from build123d import *

# Parameters (mm, degrees)
SKETCH_1_W      = 16.3
SKETCH_1_H      = 18
EXTRUDE_1_DEPTH = 10
SKETCH_3_R      = 4
EXTRUDE_2_DEPTH = 12


with BuildPart() as part:
    # Эскиз1 → Бобышка-Вытянуть1 (new body)
    with BuildSketch(Plane(origin=(0, 0, 0), x_dir=(1, 0, 0), z_dir=(0, 1, 0))):
        with Locations((8.15, 9)):
            Rectangle(SKETCH_1_W, SKETCH_1_H)
    extrude(amount=EXTRUDE_1_DEPTH)

    # Эскиз3 → Бобышка-Вытянуть2 (add)
    with BuildSketch(Plane.XZ):
        with Locations(Location((8.15, -6, 0), (0, 0, 270))):
            Circle(SKETCH_3_R)
    extrude(amount=EXTRUDE_2_DEPTH)


solid = part.part
Verification items for the finished model (mm, model axes). A direction names the side the tool comes from. Coordinates: 2 decimals unless noted, no trailing zeros. Order: outer loops, then holes, each group sorted by start corner. A loop starts at its lowest first (then second) coordinate and runs counter-clockwise, first axis right, second up. Notation, with made-up numbers: (46, 25.25) -> (104, 25.25) arc R20 ccw to (104, 56.25) -> close; hole circle Ø2 at (-5.75, 67). An arc over 180 degrees is marked (long way). Put each result on its own line as item: value. Start each with the question number.
1. Cross-section at A-A, the plane x = 8.15. Record the boundary of the cut face in (y, z).
2. Cross-section at D-D, the plane x = 2.5. Record the boundary of the cut face in (y, z), then the cut area to 3 significant figures.
3. Access from +Z, -Z, +X, -X, +Y, -Y to the whole of each face (thin tool, end or side, straight path). Record for faces 1 (the flat face through (8, -12, -6)), 2 (the cylindrical face through (12.116, -5.916, -5.479)).
4. Cross-section at C-C, the plane y = -6.5. Record the boundary of the cut face in (x, z), then the cut area to 3 significant figures.
5. Material ranges on L1, parallel to Y at x = 11.5, z = -13.25; L2, parallel to Z at x = 10, y = -6.75; L3, parallel to Z at x = 11.25, y = -5.75, recorded low to high. Write a range as [from, to].
6. Cross-section at B-B, the plane z = -6. Record the boundary of the cut face in (x, y), then the cut area to 3 significant figures.
7. Go/stop test with a flat-tipped pin: pin 1 Ø3 at (y, z) = (-7, -7.5) entering from +X. Record where the tip stops, or that it passes through.
Computed:
1. outline: (-12, -10) -> (0, -10) -> (0, -18) -> (10, -18) -> (10, 0) -> (0, 0) -> (0, -2) -> (-12, -2) -> close
2. outline: (0, -18) -> (10, -18) -> (10, 0) -> (0, 0) -> close
2. area: 180 mm2
3. face 1: +Z, -Z, +X, -X, -Y
3. face 2: -Y
4. outline: circle Ø8 at (8.15, -6)
4. area: 50.3 mm2
5. L1: [0, 10]
5. L2: [-9.55, -2.45]
5. L3: [-8.53, -3.47]
6. outline: (0, 0) -> (4.15, 0) -> (4.15, -12) -> (12.15, -12) -> (12.15, 0) -> (16.3, 0) -> (16.3, 10) -> (0, 10) -> close
6. area: 259 mm2
7. pin 1: x = 12.15
